Check sheet for the modelled part. Datum: model origin and axes. Units: mm. A direction names the side the tool comes from. Coordinates: 2 decimals unless noted, no trailing zeros. Loops run counter-clockwise (first coordinate to the right, second up) from the corner with the lowest first, then second, coordinate; pieces in that order, holes last.
```python
from build123d import *

# Parameters (mm, degrees)
SKETCH1_W           = 100
SKETCH1_H           = 25
BOSS_EXTRUDE1_DEPTH = 10
SKETCH2_R           = 1.19
SKETCH2_W           = 23.5
SKETCH2_H           = 13
CUT_EXTRUDE1_DEPTH  = 10
BOSS_EXTRUDE2_DEPTH = 10
FILLET1_R           = 10
SKETCH7_W           = 34
SKETCH7_H           = 17.658274854
BOSS_EXTRUDE3_DEPTH = 14.5
SKETCH8_W           = 23.5
SKETCH8_H           = 9.5
CUT_EXTRUDE2_DEPTH  = 21.735155199
SKETCH9_W           = 9.658274854
SKETCH9_H           = 9.5
CUT_EXTRUDE3_DEPTH  = 147.612554477
SKETCH10_R          = 2.899136991
BOSS_EXTRUDE4_DEPTH = 5
CUT_EXTRUDE4_DEPTH  = 30.5


with BuildPart() as part:
    # Sketch1 → Boss-Extrude1 (new body)
    with BuildSketch(Plane(origin=(0, 0, 0), x_dir=(1, 0, 0), z_dir=(0, 1, 0))):
        with Locations((50, 12.5)):
            Rectangle(SKETCH1_W, SKETCH1_H)
    extrude(amount=BOSS_EXTRUDE1_DEPTH)

    # Sketch2 → Cut-Extrude1 (cut)
    with BuildSketch(Plane(origin=(0, 10, 0), x_dir=(1, 0, 0), z_dir=(0, 1, 0))):
        with Locations((7.75, 12.5)):
            Circle(SKETCH2_R)
        with Locations((35.75, 12.5)):
            Circle(SKETCH2_R)
        with Locations((21.75, 12.5)):
            Rectangle(SKETCH2_W, SKETCH2_H)
    extrude(amount=-CUT_EXTRUDE1_DEPTH, mode=Mode.SUBTRACT)

    # Sketch3 → Boss-Extrude2 (add)
    with BuildSketch(Plane(origin=(0, 10, 0), x_dir=(1, 0, 0), z_dir=(0, 1, 0))):
        with BuildLine():
            add(Edge.make_bspline(
                [(100, 0), (130.91054584, 0.791905692), (151.535957226, -16.787524717)],
                knots=[0, 0, 0, 1, 1, 1], degree=2))
            add(Edge.make_bspline(
                [(100, 25), (145.583275761, 15.848400437), (151.535957226, -16.787524717)],
                knots=[0, 0, 0, 1, 1, 1], degree=2))
            Line((100, 25), (100, 0))
        make_face()
    extrude(amount=-BOSS_EXTRUDE2_DEPTH)

    # Fillet1
    fillet1_edges = [part.edges().sort_by_distance(p)[0] for p in [
        (0, 5, -25),
        (0, 5, 0),
    ]]
    fillet(fillet1_edges, radius=FILLET1_R)

    # Sketch7 → Boss-Extrude3 (add)
    with BuildSketch(Plane.XZ):
        with Locations((21.923402849, -13.093982328)):
            Rectangle(SKETCH7_W, SKETCH7_H)
    extrude(amount=BOSS_EXTRUDE3_DEPTH)

    # Sketch8 → Cut-Extrude2 (cut, through all)
    with BuildSketch(Plane.XY.offset(-4.264844901)):
        with Locations((21.673402849, -4.75)):
            Rectangle(SKETCH8_W, SKETCH8_H)
    extrude(amount=-CUT_EXTRUDE2_DEPTH, mode=Mode.SUBTRACT)

    # Sketch9 → Cut-Extrude3 (cut, through all)
    with BuildSketch(Plane.ZY.offset(-4.923402849)):
        with Locations((-13.093982328, -4.75)):
            Rectangle(SKETCH9_W, SKETCH9_H)
    extrude(amount=-CUT_EXTRUDE3_DEPTH, mode=Mode.SUBTRACT)

    # Sketch10 → Boss-Extrude4 (add)
    with BuildSketch(Plane.XZ.offset(14.5)):
        with Locations((16.5, -12.5)):
            Circle(SKETCH10_R)
    extrude(amount=BOSS_EXTRUDE4_DEPTH)

    # Sketch13 → Cut-Extrude4 (cut, through all)
    with BuildSketch(Plane(origin=(0, 10, 0), x_dir=(1, 0, 0), z_dir=(0, 1, 0))):
        with BuildLine():
            Line((40.759141507, 18.280493838), (40.759141507, 13.958351936))
            Line((40.759141507, 13.958351936), (40.759141507, 5.850917493))
            add(Edge.make_bspline(
                [(40.759141507, 5.850917493), (70.418760449, 8.670764937), (93.626937349, 6.822983821)],
                knots=[0, 0, 0, 0.76207728, 0.76207728, 0.76207728], degree=2))
            add(Edge.make_bspline(
                [(48.109032445, 18.802566203), (74.292639641, 20.065268225), (93.626937349, 6.822983821)],
                knots=[0, 0, 0, 0.932257027, 0.932257027, 0.932257027], degree=2))
            add(Edge.make_bspline(
                [(40.759141507, 18.280493838), (44.500946657, 18.577601375), (48.109032445, 18.802566203)],
                knots=[0, 0, 0, 0.044284704, 0.044284704, 0.044284704], degree=2))
        make_face()
        with BuildLine():
            add(Edge.make_bspline(
                [(79.05980568, 19.324038395), (129.368985963, 17.399904925), (141.56306601, -5.087642347)],
                knots=[0.252338304, 0.252338304, 0.252338304, 1, 1, 1], degree=2))
            add(Edge.make_bspline(
                [(79.05980568, 19.324038395), (103.573343897, 15.754713023), (122.487748371, 2.098418722)],
                knots=[0, 0, 0, 0.958850714, 0.958850714, 0.958850714], degree=2))
            add(Edge.make_bspline(
                [(122.487748371, 2.098418722), (125.30805626, 1.325368592), (128.089706455, 0.417067533)],
                knots=[0.632770601, 0.632770601, 0.632770601, 0.8750054, 0.8750054, 0.8750054], degree=2))
            add(Edge.make_bspline(
                [(128.089706455, 0.417067533), (129.541401077, -0.054077042), (130.95010952, -0.556322186)],
                knots=[0, 0, 0, 0.199498744, 0.199498744, 0.199498744], degree=2))
            add(Edge.make_bspline(
                [(130.95010952, -0.556322186), (136.602640718, -2.571612406), (141.56306601, -5.087642347)],
                knots=[0.199498744, 0.199498744, 0.199498744, 1, 1, 1], degree=2))
        make_face()
    extrude(amount=-CUT_EXTRUDE4_DEPTH, mode=Mode.SUBTRACT)


solid = part.part
```
1) Section check C-C on y = -16. Enter the section's corners in (x, z), plus the area to 3 significant figures.
Answer sheet:
outline: circle Ø5.8 at (16.5, -12.5)
area: 26.4 mm2
2) Set-up check for faces 1 (the flat face through (38.923, -10, -13)), 2 (the cylindrical face through (14.4, -17, -10.5)), 3 (the flat face through (36, -5, -8.265)), 4 (the flat face through (33.5, 5, -12)): record each of +Z, -Z, +X, -X, +Y, -Y from which the full face is reachable in a straight line by a thin tool's end or side.
Answer sheet:
face 1: +Z, -Z, +X, -Y
face 2: -Y
face 3: +X, -X
face 4: +Y
3) Section check A-A on x = 24.5. Enter the section's corners in (y, z), plus the area to 3 significant figures.
Answer sheet:
outline: (-14.5, -21.92) - (-9.5, -21.92) - (-9.5, -4.26) - (-14.5, -4.26) - close; (0, -25) - (10, -25) - (10, -19) - (0, -19) - close; (0, -6) - (10, -6) - (10, 0) - (0, 0) - close
area: 208 mm2
4) Section check B-B on y = 3.25. Give the number of separate pieces and of enclosed holes in the cut face, plus the area to 3 significant figures.
Answer sheet:
separate pieces: 1
enclosed holes: 5
area: 2,330 mm2
5) Scan lines: line 1 (Z direction, x = 35.75, y = 3); line 2 (Z direction, x = 86.5, y = 1.5); line 3 (Y direction, x = 63, z = -2.5). Record each from-to range of solid material in increasing order.
Answer sheet:
line 1: z = -25 to -13.69, -11.31 to 0
line 2: z = -25 to -18.91, -17.98 to -11.09, -7.27 to 0
line 3: y = 0 to 10
6) Depth check by flat-ended pin: pin 1 (11 mm diameter, centred on y = 4, z = -13.5, fed in from +X); pin 2 (12 mm diameter, centred on y = -12.5, z = -19, fed in from -X); pin 3 (7 mm diameter, centred on x = 16.5, y = -9.5, fed in from +Z). Enter the tip coordinate at first touch or a pass-through.
Answer sheet:
pin 1: stops at x = 137.97
pin 2: stops at x = 4.92
pin 3: stops at z = -4.26
7) Mould release check, pull along X, two halves, no side actions. Record for faces 5 (the flat face through (4.923, -10, -13)), 6 (the flat face through (33.423, -5, -6)), 7 (the flat face through (7, -5, -8.265)): +X half, -X half, draft (parallel to the pull), parting line (faces both ways), or undercut.
Answer sheet:
face 5: -X half
face 6: undercut
face 7: draft
